Autodesk Inventor part; units mm, degrees
ref_plane "YZ Plane" through (0, 0, 0) normal (1, 0, 0) x (0, 1, 0)
ref_plane "XZ Plane" through (0, 0, 0) normal (0, 1, 0) x (-1, 0, 0)
ref_plane "XY Plane" through (0, 0, 0) normal (0, 0, 1) x (1, 0, 0)
sketch "Sketch1" plane through (0, 0, 0) normal (0, 0, 1) x (1, 0, 0)
  line L0 (-36, 16) -> (36, 16)
  line L1 (36, 16) -> (36, -16)
  line L2 (36, -16) -> (-36, -16)
  line L3 (-36, -16) -> (-36, 16)
  line L4 (-36, -16) -> (36, 16) construction
  line L5 (4, 16) -> (-36, 8)
  line L6 (-36, -8) -> (4, -16)
  line L7 (4, 16) -> (4, -16) construction
  circle A0 centre (-32, 4) radius 2.5
  circle A1 centre (32, 12) radius 2.5
  point P0 (0, 0)
  point P1 (0, 0)
  dimension "d0" = 32
  dimension "d1" = 72
  dimension "d2" = 32
  dimension "d3" = 16
  dimension "d4" = 5
  dimension "d5" = 4
  dimension "d6" = 4
  dimension "d7" = 4
  dimension "d8" = 4
extrude "Extrusion1" add sketch "Sketch1" against normal blind 3.2 contours L0 L1 L2 L6 L3 L5 | A0 | A1
extrude "Extrusion2" add sketch "Sketch1" along normal blind 1.6 contours A0
pattern_linear "Rectangular Pattern1" count 5 spacing 8 along (1, 0, 0) count 2 spacing 8 along (0, -1, 0) of "Extrusion2"
extrude "Extrusion3" add sketch "Sketch1" along normal blind 1.6 contours A1
pattern_linear "Rectangular Pattern2" count 4 spacing 8 along (-1, 0, 0) count 4 spacing 8 along (0, -1, 0) of "Extrusion3"
sketch "Sketch2" plane through (0, 0, -3.2) normal (0, 0, -1) x (-1, 0, 0)
  circle A0 centre (32, 4) radius 2.5 construction
  circle A1 centre (24, 4) radius 2.5 construction
  circle A2 centre (16, 4) radius 2.5 construction
  circle A3 centre (8, 4) radius 2.5 construction
  circle A4 centre (0, 4) radius 2.5 construction
  circle A5 centre (-8, 4) radius 2.5 construction
  circle A6 centre (-16, 4) radius 2.5 construction
  circle A7 centre (-24, 4) radius 2.5 construction
  circle A8 centre (-32, 4) radius 2.5 construction
  circle A9 centre (-32, 12) radius 2.5 construction
  circle A10 centre (-24, 12) radius 2.5 construction
  circle A11 centre (-16, 12) radius 2.5 construction
  circle A12 centre (-8, 12) radius 2.5 construction
  circle A13 centre (-32, -4) radius 2.5 construction
  circle A14 centre (-24, -4) radius 2.5 construction
  circle A15 centre (-16, -4) radius 2.5 construction
  circle A16 centre (-8, -4) radius 2.5 construction
  circle A17 centre (0, -4) radius 2.5 construction
  circle A18 centre (8, -4) radius 2.5 construction
  circle A19 centre (16, -4) radius 2.5 construction
  circle A20 centre (24, -4) radius 2.5 construction
  circle A21 centre (32, -4) radius 2.5 construction
  circle A22 centre (-8, -12) radius 2.5 construction
  circle A23 centre (-16, -12) radius 2.5 construction
  circle A24 centre (-24, -12) radius 2.5 construction
  circle A25 centre (-32, -12) radius 2.5 construction
  line L0 (-34.5, -14.5) -> (-5.5, -14.5)
  line L1 (-5.5, -14.5) -> (-5.5, -6.5)
  line L2 (-5.5, -6.5) -> (34.5, -6.5)
  line L3 (34.5, -6.5) -> (34.5, 6.5)
  line L4 (34.5, 6.5) -> (-5.5, 6.5)
  line L5 (-5.5, 6.5) -> (-5.5, 14.5)
  line L6 (-5.5, 14.5) -> (-34.5, 14.5)
  line L7 (-34.5, 14.5) -> (-34.5, -14.5)
  circle A26 centre (-28, -8) radius 3.1569
  circle A27 centre (-28, -8) radius 2.3569
  circle A28 centre (-28, 0) radius 3.1569
  circle A29 centre (-28, 0) radius 2.3569
  dimension "d27" = 0.8
extrude "Extrusion4" cut sketch "Sketch2" against normal blind 2 contours L7 L6 L5 L4 L3 L2 L1 L0 | A26 | A27 | A28 | A29
extrude "Extrusion5" add sketch "Sketch2" against normal blind 2 contours A26
extrude "Extrusion6" add sketch "Sketch2" against normal blind 2 contours A28
pattern_linear "Rectangular Pattern3" count 3 spacing 8 along (-1, 0, 0) count 2 spacing 16 along (0, 1, 0) of "Extrusion5"
pattern_linear "Rectangular Pattern4" count 8 spacing 8 along (-1, 0, 0) of "Extrusion6"
properties part number "LEGO Brick 2413" material "Steel"
Design review of the part built by this model. Coordinates are the model's own, in mm. A direction names the side the tool comes from. Coordinates: 2 decimals unless noted, no trailing zeros. Loops run counter-clockwise (first coordinate to the right, second up) from the corner with the lowest first, then second, coordinate; pieces in that order, holes last.
Q1. We need section C-C on x = -12. State the section outline as (y, z) points, and give its area (3 significant figures).
Reported:
outline: (-12.8, -3.2) - (-6.5, -3.2) - (-6.5, -1.2) - (-3.16, -1.2) - (-3.16, -3.2) - (-2.36, -3.2) - (-2.36, -1.2) - (2.36, -1.2) - (2.36, -3.2) - (3.16, -3.2) - (3.16, -1.2) - (6.5, -1.2) - (6.5, -3.2) - (12.8, -3.2) - (12.8, 0) - (-12.8, 0) - close
area: 59.1 mm2
Q2. To check wall thickness, follow line 1 (Y direction, x = -12, z = -2.65); line 2 (Y direction, x = -28, z = -1.95); line 3 (X direction, y = -5.5, z = -1.4). State the ranges of each line that lie inside material, in increasing order.
Reported:
line 1: y = -12.8 to -6.5, -3.16 to -2.36, 2.36 to 3.16, 6.5 to 12.8
line 2: y = -9.6 to -6.5, -3.16 to -2.36, 2.36 to 3.16, 6.5 to 9.6
line 3: x = -36 to -34.5, 10.07 to 13.93, 18.07 to 21.93, 26.07 to 29.93, 34.5 to 36
Q3. We need section B-B on y = 12. State the section outline as (x, z) points.
Reported:
outline: (-16, -3.2) - (5.5, -3.2) - (5.5, -1.2) - (34.5, -1.2) - (34.5, -3.2) - (36, -3.2) - (36, 0) - (34.5, 0) - (34.5, 1.6) - (29.5, 1.6) - (29.5, 0) - (26.5, 0) - (26.5, 1.6) - (21.5, 1.6) - (21.5, 0) - (18.5, 0) - (18.5, 1.6) - (13.5, 1.6) - (13.5, 0) - (10.5, 0) - (10.5, 1.6) - (5.5, 1.6) - (5.5, 0) - (-16, 0) - close
Q4. For pin 1 (1.4 mm diameter, centred on x = 4, y = 0.5, fed in from -Z); pin 2 (5.5 mm diameter, centred on x = -4, y = 0, fed in from +Z); pin 3 (2 mm diameter, centred on x = -16, z = -2.5, fed in from -Y), all flat-tipped, find the tip position at first contact; note any pin that passes through.
Reported:
pin 1: stops at z = -1.2
pin 2: stops at z = 0
pin 3: stops at y = -12.2
Q5. The part is to be moulded in two halves that separate along X. For faces 4 (the face through (36, 0, -2)), 5 (the face through (21.74, -6.41, -2.21)), 6 (the face through (-17.645, 0.104, -2.214)), 7 (the face through (32, 12, 1.6)), say which applies: +X half, -X half, draft (parallel to the pull), parting line (faces both ways), or undercut.
Reported:
face 4: +X half
face 5: undercut
face 6: undercut
face 7: draft
Q6. We need section D-D on x = -4. State the section outline as (y, z) points.
Reported:
outline: (-14.4, -3.2) - (-6.5, -3.2) - (-6.5, -1.2) - (-3.16, -1.2) - (-3.16, -3.2) - (-2.36, -3.2) - (-2.36, -1.2) - (2.36, -1.2) - (2.36, -3.2) - (3.16, -3.2) - (3.16, -1.2) - (6.5, -1.2) - (6.5, -3.2) - (14.4, -3.2) - (14.4, 0) - (-14.4, 0) - close
Q7. Tool access review of faces 1 (the face through (8, -12, 1.6)), 2 (the face through (-8.846, 0.139, -2.214)), 3 (the face through (9.15, 14.22, 0.79)): name each direction out of +Z, -Z, +X, -X, +Y, -Y from which nothing blocks a thin tool from reaching the whole face with its end or side.
Reported:
face 1: +Z, +X, -X, +Y, -Y
face 2: -Z
face 3: +Z
Q8. We need section A-A on x = 32. State the section outline as (y, z) points, and give its area (3 significant figures).
Reported:
outline: (-16, -3.2) - (-14.5, -3.2) - (-14.5, -1.2) - (14.5, -1.2) - (14.5, -3.2) - (16, -3.2) - (16, 0) - (14.5, 0) - (14.5, 1.6) - (9.5, 1.6) - (9.5, 0) - (6.5, 0) - (6.5, 1.6) - (1.5, 1.6) - (1.5, 0) - (-1.5, 0) - (-1.5, 1.6) - (-6.5, 1.6) - (-6.5, 0) - (-9.5, 0) - (-9.5, 1.6) - (-14.5, 1.6) - (-14.5, 0) - (-16, 0) - close
area: 76.4 mm2
